Input: part model. Units: mm. Frame: model coordinates. A direction names the side the tool comes from. Coordinates: 2 decimals unless noted, no trailing zeros. Loops run counter-clockwise (first coordinate to the right, second up) from the corner with the lowest first, then second, coordinate; pieces in that order, holes last. Notation, with made-up numbers: (-23, 59.5) - (-7, 59.5) arc R16 ccw to (-7, 83.5) - close; hole circle Ø11 at (81, -11.75). An arc over 180 degrees is marked (long way). Use one line per item in the form item = value.
from build123d import *

# Parameters (mm, degrees)
F1_DEPTH = 514.35
F3_DEPTH = 25.4


with BuildPart() as f1:
    # F0 (on Front) → F1 (new body, symmetric)
    with BuildSketch(Plane.XZ):
        with BuildLine():
            Line((0, 6.35), (-609.6, 6.35))
            Line((-609.6, 6.35), (-609.6, 38.1))
            Line((-609.6, 38.1), (-615.95, 38.1))
            Line((-615.95, 38.1), (-615.95, 0))
            Line((-615.95, 0), (0, 0))
            Line((0, 0), (0, -50.8))
            Line((0, -50.8), (6.35, -50.8))
            Line((6.35, -50.8), (6.35, 0))
            ThreePointArc((6.35, 0), (4.4901280605, 4.4901280605), (0, 6.35))
        make_face()
    extrude(amount=F1_DEPTH, both=True)

    # F2 (on face) → F3 (cut)
    with BuildSketch(Plane.XY.offset(6.35)):
        with BuildLine():
            Line((-114.3, 342.9), (-469.9, 342.9))
            ThreePointArc((-469.9, 342.9), (-505.8210244843, 328.0210244843), (-520.7, 292.1))
            Line((-520.7, 292.1), (-520.7, -406.4))
            ThreePointArc((-520.7, -406.4), (-505.8210244843, -442.3210244843), (-469.9, -457.2))
            Line((-469.9, -457.2), (-114.3, -457.2))
            ThreePointArc((-114.3, -457.2), (-78.3789755157, -442.3210244843), (-63.5, -406.4))
            Line((-63.5, -406.4), (-63.5, 292.1))
            ThreePointArc((-63.5, 292.1), (-78.3789755157, 328.0210244843), (-114.3, 342.9))
        make_face()
    extrude(amount=-F3_DEPTH, mode=Mode.SUBTRACT)


solid = f1.part
Q1. Set-up query: faces 1 (the flat face through (-615.95, -7, 19)), 2 (the cylindrical face through (-505.424, 328.414, 3.219)), 3 (the flat face through (0, -7, -25)), 4 (the flat face through (-609.6, -7, 22)), 5 (the flat face through (-306, -514.35, 4)). Return all of +Z, -Z, +X, -X, +Y, -Y with unobstructed straight access to the full face (end or side cutting, diameter ignored); none if empty.
Check values:
face_1 = +Z, -Z, -X, +Y, -Y
face_2 = +Z, -Z
face_3 = -Z, -X, +Y, -Y
face_4 = +Z, +X, +Y, -Y
face_5 = +Z, -Z, +X, -X, -Y
Q2. Cut plane A-A, the plane x = -164.5. Return loops of the section in (y, z).
Check values:
outline = (-514.35, 0) - (-457.2, 0) - (-457.2, 6.35) - (-514.35, 6.35) - close; (342.9, 0) - (514.35, 0) - (514.35, 6.35) - (342.9, 6.35) - close
Q3. Pull-direction query (X, two-part tool) for faces 6 (the cylindrical face through (-77.986, 327.624, 3.219)), 7 (the cylindrical face through (-506.214, -441.924, 3.219)), 8 (the flat face through (6.35, -7, -26)), 9 (the flat face through (-571, -7, 6.35)); classes: pulls with the +X half, pulls with the -X half, needs draft (parallel to the pull), parting line crosses it, or undercut.
Check values:
face_6 = undercut
face_7 = undercut
face_8 = pulls with the +X half
face_9 = needs draft
Q4. Cut plane C-C, the plane y = 387.5. Return loops of the section in (x, z), then the cut area to 3 significant figures.
Check values:
outline = (-615.95, 0) - (0, 0) - (0, -50.8) - (6.35, -50.8) - (6.35, 0) arc R6.35 ccw to (0, 6.35) - (-609.6, 6.35) - (-609.6, 38.1) - (-615.95, 38.1) - close
area = 4,470 mm²
Q5. Cut plane B-B, the plane y = -117.5. Return loops of the section in (x, z), then the cut area to 3 significant figures.
Check values:
outline = (-615.95, 0) - (-520.7, 0) - (-520.7, 6.35) - (-609.6, 6.35) - (-609.6, 38.1) - (-615.95, 38.1) - close; (-63.5, 0) - (0, 0) - (0, -50.8) - (6.35, -50.8) - (6.35, 0) arc R6.35 ccw to (0, 6.35) - (-63.5, 6.35) - close
area = 1,560 mm²
Q6. Ray query, line 1 along X through (y, z) = (127, 1.5); line 2 along X through (y, z) = (-307, 14.5); line 3 along X through (y, z) = (280, -47). Return the intervals inside material, ascending. Write a range as [from, to].
Check values:
line_1 = [-615.95, -520.7], [-63.5, 6.17]
line_2 = [-615.95, -609.6]
line_3 = [0, 6.35]
Q7. First-contact query: P1, Ø1.9, axis at y = -177.5, z = 3, coming from the +X side; P2, Ø1, axis at x = -515, y = 385.5, coming from the +Z side; P3, Ø1.5, axis at y = 104.5, z = -21, coming from the -X side. Flat tips, straight axial feed; report the tip coordinate or a pass-through.
Check values:
P1 = 6.01
P2 = 6.35
P3 = 0
Q8. Cut plane D-D, the plane x = -499.5. Return loops of the section in (y, z).
Check values:
outline = (-514.35, 0) - (-447.69, 0) - (-447.69, 6.35) - (-514.35, 6.35) - close; (333.39, 0) - (514.35, 0) - (514.35, 6.35) - (333.39, 6.35) - close
